from build123d import *

# Parameters (mm, degrees)
SKETCH1_W           = 38.1
SKETCH1_H           = 25.4
BOSS_EXTRUDE1_DEPTH = 76.2
SKETCH2_R           = 3.302
CUT_EXTRUDE1_DEPTH  = 80.565271947
SKETCH3_R           = 3.302
CUT_EXTRUDE2_DEPTH  = 83.55
SKETCH5_R           = 0.889
CUT_EXTRUDE3_DEPTH  = 12.7
CUT_EXTRUDE4_START  = -12.7
SKETCH6_R           = 0.889
CUT_EXTRUDE4_DEPTH  = 12.7


with BuildPart() as part:
    # Sketch1 → Boss-Extrude1 (new body)
    with BuildSketch(Plane.XY):
        Rectangle(SKETCH1_W, SKETCH1_H)
    extrude(amount=BOSS_EXTRUDE1_DEPTH)

    # Sketch2 → Cut-Extrude1 (cut, through all)
    with BuildSketch(Plane.XY.offset(76.2)):
        Circle(SKETCH2_R)
    extrude(amount=-CUT_EXTRUDE1_DEPTH, mode=Mode.SUBTRACT)

    # Sketch3 → Cut-Extrude2 (cut, through all)
    with BuildSketch(Plane(origin=(0, 12.7, 0), x_dir=(1, 0, 0), z_dir=(0, 1, 0))):
        with Locations(Location((-11.1125, -25.4, 0), (0, 0, 180))):
            Circle(SKETCH3_R)
        with Locations(Location((11.1125, -25.4, 0), (0, 0, 180))):
            Circle(SKETCH3_R)
        with Locations(Location((-11.1125, -50.8, 0), (0, 0, 180))):
            Circle(SKETCH3_R)
        with Locations(Location((11.1125, -50.8, 0), (0, 0, 180))):
            Circle(SKETCH3_R)
    extrude(amount=-CUT_EXTRUDE2_DEPTH, mode=Mode.SUBTRACT)

    # Sketch5 → Cut-Extrude3 (cut)
    with BuildSketch(Plane(origin=(19.05, 0, 0), x_dir=(0, 0, -1), z_dir=(1, 0, 0))):
        with Locations((-38.1, 9.525)):
            Circle(SKETCH5_R)
    extrude(amount=-CUT_EXTRUDE3_DEPTH, mode=Mode.SUBTRACT)

    # Sketch6 → Cut-Extrude4 (cut)
    with BuildSketch(Plane.ZY.offset(19.05).offset(CUT_EXTRUDE4_START)):
        with Locations(Location((38.1, 9.525, 0), (0, 0, 180))):
            Circle(SKETCH6_R)
    extrude(amount=CUT_EXTRUDE4_DEPTH, mode=Mode.SUBTRACT)


solid = part.part
Input: part model. Units: mm. Frame: model coordinates. A direction names the side the tool comes from. Round coordinates to 2 decimals unless told otherwise and drop trailing zeros. Order: outer loops, then holes, each group sorted by start corner. A loop starts at its lowest first (then second) coordinate and runs counter-clockwise, first axis right, second up. Notation, with made-up numbers: (2, 42) - (56, 42) arc R38 cw to (56, 81) - close; hole circle Ø4 at (-33, -9.75). An arc over 180 degrees is marked (long way). Answer as a JSON object with one key per item and string values. Group by question number.
(1) Cut plane A-A (z = 50.8). Return loops of the section in (x, y), then the cut area to 3 significant figures.
(2) Cut plane D-D (z = 38.1). Return loops of the section in (x, y).
(3) Material intervals for probe 1 along X at (y, z) = (8.75, 50.5); probe 2 along Y at (x, z) = (0, 39); probe 3 along X at (y, z) = (3.5, 27.5), sorted ascending. Write a range as from..to.
(4) Draft query along Y for faces 4 (the face through (-10.683, 0.178, 54.074)), 5 (the face through (3.05, -1.26, 38.63)), 6 (the face through (-6.35, 10, 38)), 7 (the face through (0, -12.7, 38)). Return one class per face: released by +Y, released by -Y, zero draft, split by the parting line, or undercut.
(5) Reachability of faces 1 (the face through (12.79, 9.56, 38.99)), 2 (the face through (-12.611, 10.066, 38.805)), 3 (the face through (-19.05, 0, 38)) from +Z, -Z, +X, -X, +Y, -Y: full face, straight path, thin tool, end or side. Return the list, or none.
(6) Pin query (flat end, axial travel): P1, Ø10.5, axis at x = -11.11, z = 25.4, coming from the +Y side; P2, Ø6, axis at x = 0, y = 0, coming from the +Z side; P3, Ø1.1, axis at y = 9.525, z = 38.1, coming from the -X side; P4, Ø0.5, axis at y = 9.5, z = 38.5, coming from the +X side. Return the tip coordinate at first contact, or that it passes through.
(7) Cut plane B-B (y = 0). Return loops of the section in (x, z), then the cut area to 3 significant figures.
(8) Cut plane C-C (x = 0). Return loops of the section in (y, z), then the cut area to 3 significant figures.
Here are the results:
{
 "1": {"outline": "(-19.05, -12.7) - (-14.41, -12.7) - (-14.41, 12.7) - (-19.05, 12.7) - close; (-7.81, -12.7) - (7.81, -12.7) - (7.81, 12.7) - (-7.81, 12.7) - close; (14.41, -12.7) - (19.05, -12.7) - (19.05, 12.7) - (14.41, 12.7) - close; hole circle Ø6.6 at (0, 0)", "area": "598 mm^2"},
 "2": {"outline": "(-19.05, -12.7) - (19.05, -12.7) - (19.05, 8.64) - (6.35, 8.64) - (6.35, 10.41) - (19.05, 10.41) - (19.05, 12.7) - (-19.05, 12.7) - (-19.05, 10.41) - (-6.35, 10.41) - (-6.35, 8.64) - (-19.05, 8.64) - close; hole circle Ø6.6 at (0, 0)"},
 "3": {"probe 1": "x = -19.05..-14.4, -7.82..7.82, 14.4..19.05", "probe 2": "y = -12.7..-3.3, 3.3..12.7", "probe 3": "x = -19.05..-13.66, -8.56..8.56, 13.66..19.05"},
 "4": {"face 4": "zero draft", "face 5": "undercut", "face 6": "undercut", "face 7": "released by -Y"},
 "5": {"face 1": "+X", "face 2": "-X", "face 3": "+Z, -Z, -X, +Y, -Y"},
 "6": {"P1": "stops at y = 12.7", "P2": "passes through", "P3": "stops at x = -6.35", "P4": "stops at x = 6.35"},
 "7": {"outline": "(-19.05, 0) - (-3.3, 0) - (-3.3, 76.2) - (-19.05, 76.2) - close; (3.3, 0) - (19.05, 0) - (19.05, 76.2) - (3.3, 76.2) - close; hole circle Ø6.6 at (-11.11, 25.4); hole circle Ø6.6 at (-11.11, 50.8); hole circle Ø6.6 at (11.11, 25.4); hole circle Ø6.6 at (11.11, 50.8)", "area": "2,260 mm^2"},
 "8": {"outline": "(-12.7, 0) - (-3.3, 0) - (-3.3, 76.2) - (-12.7, 76.2) - close; (3.3, 0) - (12.7, 0) - (12.7, 76.2) - (3.3, 76.2) - close", "area": "1,430 mm^2"}
}
